Verification items for the finished model (mm, model axes). A direction names the side the tool comes from. Round coordinates to 2 decimals unless told otherwise and drop trailing zeros. Loops run counter-clockwise (first coordinate to the right, second up) from the corner with the lowest first, then second, coordinate; pieces in that order, holes last. Notation, with made-up numbers: (56.25, 69.5) -> (63.25, 69.5) arc R5 ccw to (63.25, 77.5) -> close; hole circle Ø10 at (-2, 9.5). An arc over 180 degrees is marked (long way). Use CSV: the item, a comma, the result in double quotes. Start each with the question number.
```python
from build123d import *

# Parameters (mm, degrees)
F0_W     = 108.2608737051
F0_H     = 38.8043485582
F1_DEPTH = 25


with BuildPart() as f1:
    # F0 (on Top) → F1 (new body)
    with BuildSketch(Plane.XY):
        with Locations((0.1630429178, -7.6630432159)):
            Rectangle(F0_W, F0_H)
        with BuildLine():
            add(Edge.make_bspline(
                [(-1.4969709304, -10.405910604), (-0.3763300382, -11.5841545327), (-0.3763300382, -13.3698486647)],
                knots=[0, 0, 0, 1, 1, 1], degree=2))
            add(Edge.make_bspline(
                [(-0.3763300382, -13.3698486647), (-0.3763300382, -15.8729624333), (-2.2405737654, -17.2318704311)],
                knots=[0, 0, 0, 1, 1, 1], degree=2))
            add(Edge.make_bspline(
                [(-2.2405737654, -17.2318704311), (-4.1048174927, -18.5907784289), (-7.4772134487, -18.5907784289)],
                knots=[0, 0, 0, 1, 1, 1], degree=2))
            add(Edge.make_bspline(
                [(-7.4772134487, -18.5907784289), (-11.043365073, -18.5907784289), (-13.0385247923, -17.4596642573)],
                knots=[0, 0, 0, 1, 1, 1], degree=2))
            Line((-13.0385247923, -17.4596642573), (-13.0385247923, -14.9408405697))
            add(Edge.make_bspline(
                [(-13.0385247923, -14.9408405697), (-11.7450747906, -15.5954205301), (-10.2657240801, -15.9698402674)],
                knots=[0, 0, 0, 1, 1, 1], degree=2))
            add(Edge.make_bspline(
                [(-10.2657240801, -15.9698402674), (-8.7863733695, -16.3442600048), (-7.4091371328, -16.3442600048)],
                knots=[0, 0, 0, 1, 1, 1], degree=2))
            add(Edge.make_bspline(
                [(-7.4091371328, -16.3442600048), (-5.2830614214, -16.3442600048), (-4.1388556506, -15.6661151658)],
                knots=[0, 0, 0, 1, 1, 1], degree=2))
            add(Edge.make_bspline(
                [(-4.1388556506, -15.6661151658), (-2.9946498798, -14.9879703268), (-2.9946498798, -13.5950241711)],
                knots=[0, 0, 0, 1, 1, 1], degree=2))
            add(Edge.make_bspline(
                [(-2.9946498798, -13.5950241711), (-2.9946498798, -12.5476962344), (-3.900588545, -11.8040933994)],
                knots=[0, 0, 0, 1, 1, 1], degree=2))
            add(Edge.make_bspline(
                [(-3.900588545, -11.8040933994), (-4.8065272102, -11.0604905644), (-7.4457936106, -10.0445824658)],
                knots=[0, 0, 0, 1, 1, 1], degree=2))
            add(Edge.make_bspline(
                [(-7.4457936106, -10.0445824658), (-9.9489073792, -9.1124606022), (-11.0040902754, -8.4159875243)],
                knots=[0, 0, 0, 1, 1, 1], degree=2))
            add(Edge.make_bspline(
                [(-11.0040902754, -8.4159875243), (-12.0592731716, -7.7195144465), (-12.5750821804, -6.8371406598)],
                knots=[0, 0, 0, 1, 1, 1], degree=2))
            add(Edge.make_bspline(
                [(-12.5750821804, -6.8371406598), (-13.0908911892, -5.9547668732), (-13.0908911892, -4.7293931873)],
                knots=[0, 0, 0, 1, 1, 1], degree=2))
            add(Edge.make_bspline(
                [(-13.0908911892, -4.7293931873), (-13.0908911892, -2.53524116), (-11.3051970572, -1.2653560368)],
                knots=[0, 0, 0, 1, 1, 1], degree=2))
            add(Edge.make_bspline(
                [(-11.3051970572, -1.2653560368), (-9.5195029252, 0.0045290864), (-6.414175593, 0.0045290864)],
                knots=[0, 0, 0, 1, 1, 1], degree=2))
            add(Edge.make_bspline(
                [(-6.414175593, 0.0045290864), (-3.5183138482, 0.0045290864), (-0.7481314557, -1.1737148424)],
                knots=[0, 0, 0, 1, 1, 1], degree=2))
            Line((-0.7481314557, -1.1737148424), (-1.7169097971, -3.3835767887))
            add(Edge.make_bspline(
                [(-1.7169097971, -3.3835767887), (-4.413779234, -2.2734091759), (-6.6079312613, -2.2734091759)],
                knots=[0, 0, 0, 1, 1, 1], degree=2))
            add(Edge.make_bspline(
                [(-6.6079312613, -2.2734091759), (-8.5402513044, -2.2734091759), (-9.522121245, -2.8782410593)],
                knots=[0, 0, 0, 1, 1, 1], degree=2))
            add(Edge.make_bspline(
                [(-9.522121245, -2.8782410593), (-10.5039911856, -3.4830729427), (-10.5039911856, -4.5461107984)],
                knots=[0, 0, 0, 1, 1, 1], degree=2))
            add(Edge.make_bspline(
                [(-10.5039911856, -4.5461107984), (-10.5039911856, -5.2687670747), (-10.134808088, -5.7741028041)],
                knots=[0, 0, 0, 1, 1, 1], degree=2))
            add(Edge.make_bspline(
                [(-10.134808088, -5.7741028041), (-9.7656249903, -6.2794385336), (-8.9487091997, -6.7376445058)],
                knots=[0, 0, 0, 1, 1, 1], degree=2))
            add(Edge.make_bspline(
                [(-8.9487091997, -6.7376445058), (-8.1317934091, -7.1958504781), (-5.8067253898, -8.0651326656)],
                knots=[0, 0, 0, 1, 1, 1], degree=2))
            add(Edge.make_bspline(
                [(-5.8067253898, -8.0651326656), (-2.6176118226, -9.2276666752), (-1.4969709304, -10.405910604)],
                knots=[0, 0, 0, 1, 1, 1], degree=2))
        make_face(mode=Mode.SUBTRACT)
        with BuildLine():
            Line((24.419158862, -0.3253792137), (27.1683946958, -0.3253792137))
            Line((27.1683946958, -0.3253792137), (27.1683946958, -11.9611925899))
            add(Edge.make_bspline(
                [(27.1683946958, -11.9611925899), (27.1683946958, -14.1553446172), (28.1659745554, -15.2340923919)],
                knots=[0, 0, 0, 1, 1, 1], degree=2))
            add(Edge.make_bspline(
                [(28.1659745554, -15.2340923919), (29.1635544151, -16.3128401667), (31.2896301265, -16.3128401667)],
                knots=[0, 0, 0, 1, 1, 1], degree=2))
            add(Edge.make_bspline(
                [(31.2896301265, -16.3128401667), (34.1069422761, -16.3128401667), (35.4056289175, -14.7758864197)],
                knots=[0, 0, 0, 1, 1, 1], degree=2))
            add(Edge.make_bspline(
                [(35.4056289175, -14.7758864197), (36.704315559, -13.2389326726), (36.704315559, -9.7513306436)],
                knots=[0, 0, 0, 1, 1, 1], degree=2))
            Line((36.704315559, -9.7513306436), (36.704315559, -0.3253792137))
            Line((36.704315559, -0.3253792137), (39.4221315546, -0.3253792137))
            Line((39.4221315546, -0.3253792137), (39.4221315546, -18.2608701289))
            Line((39.4221315546, -18.2608701289), (37.1808497702, -18.2608701289))
            Line((37.1808497702, -18.2608701289), (36.7881017939, -15.8572525143))
            Line((36.7881017939, -15.8572525143), (36.6414758828, -15.8572525143))
            add(Edge.make_bspline(
                [(36.6414758828, -15.8572525143), (35.8088501731, -17.1821223541), (34.3268811428, -17.8864503915)],
                knots=[0, 0, 0, 1, 1, 1], degree=2))
            add(Edge.make_bspline(
                [(34.3268811428, -17.8864503915), (32.8449121124, -18.5907784289), (30.9440119074, -18.5907784289)],
                knots=[0, 0, 0, 1, 1, 1], degree=2))
            add(Edge.make_bspline(
                [(30.9440119074, -18.5907784289), (27.6711121054, -18.5907784289), (26.0451354837, -17.035496443)],
                knots=[0, 0, 0, 1, 1, 1], degree=2))
            add(Edge.make_bspline(
                [(26.0451354837, -17.035496443), (24.419158862, -15.4802144571), (24.419158862, -12.0606887439)],
                knots=[0, 0, 0, 1, 1, 1], degree=2))
            Line((24.419158862, -12.0606887439), (24.419158862, -0.3253792137))
        make_face(mode=Mode.SUBTRACT)
        Polygon((-14.8242189243, -18.2608701289), (-17.7043707501, -18.2608701289), (-20.6840187299, -10.6520326691), (-30.27230599, -10.6520326691), (-33.215297492, -18.2608701289), (-36.0326096416, -18.2608701289), (-26.5752383736, 5.7648327379), (-24.2344604352, 5.7648327379), align=None, mode=Mode.SUBTRACT)
        with BuildLine():
            Line((19.0358932677, -18.2608701289), (16.318077272, -18.2608701289))
            Line((16.318077272, -18.2608701289), (16.318077272, -6.6564765908))
            add(Edge.make_bspline(
                [(16.318077272, -6.6564765908), (16.318077272, -4.4675612032), (15.3204974124, -3.3861951086)],
                knots=[0, 0, 0, 1, 1, 1], degree=2))
            add(Edge.make_bspline(
                [(15.3204974124, -3.3861951086), (14.3229175527, -2.304829014), (12.1916052016, -2.304829014)],
                knots=[0, 0, 0, 1, 1, 1], degree=2))
            add(Edge.make_bspline(
                [(12.1916052016, -2.304829014), (9.3638197727, -2.304829014), (8.0625148114, -3.8444010808)],
                knots=[0, 0, 0, 1, 1, 1], degree=2))
            add(Edge.make_bspline(
                [(8.0625148114, -3.8444010808), (6.7612098501, -5.3839731477), (6.7612098501, -8.8820484561)],
                knots=[0, 0, 0, 1, 1, 1], degree=2))
            Line((6.7612098501, -8.8820484561), (6.7612098501, -18.2608701289))
            Line((6.7612098501, -18.2608701289), (4.0433938545, -18.2608701289))
            Line((4.0433938545, -18.2608701289), (4.0433938545, 7.2049086508))
            Line((4.0433938545, 7.2049086508), (6.7612098501, 7.2049086508))
            Line((6.7612098501, 7.2049086508), (6.7612098501, -0.5034249629))
            add(Edge.make_bspline(
                [(6.7612098501, -0.5034249629), (6.7612098501, -1.8963711187), (6.630293858, -2.8127830632)],
                knots=[0, 0, 0, 1, 1, 1], degree=2))
            Line((6.630293858, -2.8127830632), (6.7926296882, -2.8127830632))
            add(Edge.make_bspline(
                [(6.7926296882, -2.8127830632), (7.5938355597, -1.5193330615), (9.0758045901, -0.7757302265)],
                knots=[0, 0, 0, 1, 1, 1], degree=2))
            add(Edge.make_bspline(
                [(9.0758045901, -0.7757302265), (10.5577736204, -0.0321273914), (12.4534371858, -0.0321273914)],
                knots=[0, 0, 0, 1, 1, 1], degree=2))
            add(Edge.make_bspline(
                [(12.4534371858, -0.0321273914), (15.7420469069, -0.0321273914), (17.3889700873, -1.5952643369)],
                knots=[0, 0, 0, 1, 1, 1], degree=2))
            add(Edge.make_bspline(
                [(17.3889700873, -1.5952643369), (19.0358932677, -3.1584012823), (19.0358932677, -6.5622170765)],
                knots=[0, 0, 0, 1, 1, 1], degree=2))
            Line((19.0358932677, -6.5622170765), (19.0358932677, -18.2608701289))
        make_face(mode=Mode.SUBTRACT)
    extrude(amount=F1_DEPTH)


solid = f1.part
```
Q1. Tool access check on faces 3 (the face through (-1, -7, 0)), 4 (the face through (5, 7.205, 12)). Record the directions out of +Z, -Z, +X, -X, +Y, -Y that give a thin tool (end or side, any length) a straight path to the whole face; none if there is none.
Q2. Cross-section at B-B (x = -35). Record the boundary of the cut face in (y, z).
Q3. Depth check by flat-ended pin: pin 1 Ø12 at (x, y) = (27, -5) entering from -Z. Enter the tip coordinate at first touch or a pass-through.
Q4. Cross-section at A-A (y = 4). Record the boundary of the cut face in (x, z).
Q5. Release check for a two-part mould opening along X. For faces 1 (the face through (-31.37, -6.42, 12.32)), 2 (the face through (-1, 11.739, 12)) record: +X half, -X half, draft (parallel to the pull), parting line (faces both ways), or undercut.
Q6. Thickness scan on L1, parallel to X at y = 2, z = 13.5; L2, parallel to Y at x = -9, z = 3.75; L3, parallel to Y at x = 4.5, z = 9. Record the ranges inside material, lowest first. Write a range as from..to.
Q7. Cross-section at C-C (z = 8). State how many separate pieces and enclosed holes the cut face has, and give its area (3 significant figures).
Answer list:
1,face 3,"-Z, +X, -X, +Y, -Y"
1,face 4,"+Z, -Z"
2,outline,"(-27.07, 0) -> (-18.26, 0) -> (-18.26, 25) -> (-27.07, 25) -> close; (-15.64, 0) -> (11.74, 0) -> (11.74, 25) -> (-15.64, 25) -> close"
3,pin 1,"stops at z = 0"
4,outline,"(-53.97, 0) -> (-27.27, 0) -> (-27.27, 25) -> (-53.97, 25) -> close; (-23.54, 0) -> (4.04, 0) -> (4.04, 25) -> (-23.54, 25) -> close; (6.76, 0) -> (54.29, 0) -> (54.29, 25) -> (6.76, 25) -> close"
5,face 1,"undercut"
5,face 2,"draft"
6,L1,"x = -53.97..-28.06, -22.76..4.04, 6.76..54.29"
6,L2,"y = -27.07..-18.53, -16.22..-9.43, -6.71..-2.62, -0.27..11.74"
6,L3,"y = -27.07..-18.26, 7.2..11.74"
7,separate pieces,"1"
7,enclosed holes,"4"
7,area,"3,660 mm2"
